Check sheet for the modelled part. Datum: model origin and axes. Units: mm. Round coordinates to 2 decimals unless told otherwise and drop trailing zeros. Loops run counter-clockwise (first coordinate to the right, second up) from the corner with the lowest first, then second, coordinate; pieces in that order, holes last. Notation, with made-up numbers: (53, 20) -> (99, 20) arc R18 cw to (99, 31) -> close; hole circle Ø10 at (-29, 29). An arc over 180 degrees is marked (long way). Return JSON: item names as keys, results as strings.
from build123d import *

# Parameters (mm, degrees)
F1_DEPTH = 168.3612558991
F2_R     = 248.5661214156
F3_DEPTH = 465.3762876987


with BuildPart() as f1:
    # F0 (on Top) → F1 (new body)
    with BuildSketch(Plane.XY):
        with BuildLine():
            ThreePointArc((8.0145221095, 246.9024653068), (32.3936051962, 300.7875887608), (81.0866635692, 334.3574009155))
            ThreePointArc((81.0866635692, 334.3574009155), (-53.0382414334, 362.1621199722), (-82.0123294419, 228.2849569913))
            ThreePointArc((-82.0123294419, 228.2849569913), (-38.1519563911, 243.1694146609), (8.0145221095, 246.9024653068))
        make_face()
    extrude(amount=F1_DEPTH)


with BuildPart() as f3:
    # F2 (on Front) → F3 (new body)
    with BuildSketch(Plane.XZ):
        with Locations((209.6148729324, -50.4343286157)):
            Circle(F2_R)
    extrude(amount=-F3_DEPTH)


with BuildPart() as f1_1:
    add(f1.part)

    # F4: intersect F3
    add(f3.part, mode=Mode.INTERSECT)


solid = f1_1.part
Q1. Section check A-A (z = 21). Record the boundary of the cut face in (x, y), then the cut area to 3 significant figures.
Results list:
{"outline": "(-28.47, 244.91) arc R188.39 cw to (8.01, 246.9) arc R110.4 cw to (81.09, 334.36) arc R97.28 ccw to (-28.47, 373.63) -> close", "area": "8,860 mm^2"}
Q2. Section check D-D (z = 124.5). Record the boundary of the cut face in (x, y).
Results list:
{"outline": "(33.03, 301.54) arc R110.4 cw to (81.09, 334.36) arc R97.28 ccw to (33.03, 372.11) -> close"}
Q3. Go/stop test with flat-tipped pins: pin 1 (1 mm diameter, centred on y = 322, z = 44.5, fed in from -X); pin 2 (12 mm diameter, centred on y = 359.5, z = 135.5, fed in from +X); pin 3 (2 mm diameter, centred on y = 363.5, z = 70, fed in from -X). Record where each tip stops, or that it passes through.
Results list:
{"pin 1": "x = -20.31", "pin 2": "x = 64.43", "pin 3": "x = -8.38"}
Q4. Section check B-B (x = 65). Record the boundary of the cut face in (y, z).
Results list:
{"outline": "(327.33, 0) -> (352.99, 0) -> (352.99, 151.73) -> (327.33, 151.73) -> close"}
Q5. Material ranges on line 1 (Y direction, x = 33, z = 43); line 2 (X direction, y = 280, z = 69); line 3 (Y direction, x = 38.5, z = 13), recorded low to high.
Results list:
{"line 1": "301.51 to 372.12", "line 2": "-8.38 to 18.68", "line 3": "307.51 to 369.95"}
Q6. Section check C-C (y = 366.5). Record the boundary of the cut face in (x, z).
Results list:
{"outline": "(-33.78, 0) -> (45.68, 0) -> (45.68, 136.41) arc R248.57 ccw to start"}
Q7. Draft check along X on faces 1 (the flat face through (10, 327, 0)), 2 (the cylindrical face through (-8.6, 246.877, 36.268)), 3 (the cylindrical face through (31.859, 300.142, 61.989)), 4 (the cylindrical face through (-4.83, 310.06, 75.26)). Enter one of: released by +X, released by -X, zero draft, split by the parting line, or undercut.
Results list:
{"face 1": "zero draft", "face 2": "undercut", "face 3": "released by +X", "face 4": "released by -X"}
